```python
from build123d import *

# Parameters (mm, degrees)
F0_W     = 50
F0_H     = 50
F1_DEPTH = 30
F2_R     = 4.45
F3_DEPTH = 30
F3_TAPER = -2
F4_W     = 50
F4_H     = 70
F5_DEPTH = 10


with BuildPart() as f1:
    # F0 (on Top) → F1 (new body)
    with BuildSketch(Plane.XY):
        Rectangle(F0_W, F0_H)
    extrude(amount=F1_DEPTH)

    # F2 (on Top) → F3 (cut)
    with BuildSketch(Plane.XY):
        with Locations((10, 10)):
            Circle(F2_R)
        with Locations((-10, 10)):
            Circle(F2_R)
        with Locations((10, -10)):
            Circle(F2_R)
        with Locations((-10, -10)):
            Circle(F2_R)
    extrude(amount=F3_DEPTH, taper=F3_TAPER, mode=Mode.SUBTRACT)

    # F4 (on Top) → F5 (join)
    with BuildSketch(Plane.XY):
        Rectangle(F4_W, F4_H)
    extrude(amount=-F5_DEPTH)


solid = f1.part
```
Geometry check sheet. Reference: the model listing, model coordinates, mm. A direction names the side the tool comes from. Coordinates: 2 decimals unless noted, no trailing zeros. Order: outer loops, then holes, each group sorted by start corner. A loop starts at its lowest first (then second) coordinate and runs counter-clockwise, first axis right, second up.
Q1. Tool access check on faces 1 (the face through (0, 0, -10)), 2 (the face through (0, 35, -5)), 3 (the face through (0, -30, 0)), 4 (the face through (0, 30, 0)), 5 (the face through (10, -10, 0)). Record the directions out of +Z, -Z, +X, -X, +Y, -Y that give a thin tool (end or side, any length) a straight path to the whole face; none if there is none.
Reply:
face 1: -Z, +X, -X, +Y, -Y
face 2: +Z, -Z, +X, -X, +Y
face 3: +Z, +X, -X, -Y
face 4: +Z, +X, -X, +Y
face 5: +Z
Q2. Thickness scan on probe 1 along Y at (x, z) = (-10, 27); probe 2 along Y at (x, z) = (12.5, 21.5); probe 3 along X at (y, z) = (-5.5, 28). Record the ranges inside material, lowest first.
Reply:
probe 1: y = -25 to -15.39, -4.61 to 4.61, 15.39 to 25
probe 2: y = -25 to -14.56, -5.44 to 5.44, 14.56 to 25
probe 3: x = -25 to -13.03, -6.97 to 6.97, 13.03 to 25
Q3. Sectioned sample at A-A on x = 0.5. Record the cut outline in (y, z).
Reply:
outline: (-35, -10) - (35, -10) - (35, 0) - (25, 0) - (25, 30) - (-25, 30) - (-25, 0) - (-35, 0) - close
Q4. Sectioned sample at B-B on z = 26. Record the cut outline in (x, y), and give its area (3 significant figures).
Reply:
outline: (-25, -25) - (25, -25) - (25, 25) - (-25, 25) - close; hole circle Ø10.72 at (-10, -10); hole circle Ø10.72 at (-10, 10); hole circle Ø10.72 at (10, -10); hole circle Ø10.72 at (10, 10)
area: 2,140 mm2
Q5. Sectioned sample at D-D on x = -10. Record the cut outline in (y, z), and give its area (3 significant figures).
Reply:
outline: (-35, -10) - (35, -10) - (35, 0) - (25, 0) - (25, 30) - (15.5, 30) - (14.45, 0) - (5.55, 0) - (4.5, 30) - (-4.5, 30) - (-5.55, 0) - (-14.45, 0) - (-15.5, 30) - (-25, 30) - (-25, 0) - (-35, 0) - close
area: 1,600 mm2
Q6. Draft check along X on faces 6 (the face through (25, 0, 10)), 7 (the face through (-5.25, -8.5, 15.21)), 8 (the face through (10, 10, 0)), 9 (the face through (0, -35, -5)). Enter one of: released by +X, released by -X, zero draft, split by the parting line, or undercut.
Reply:
face 6: released by +X
face 7: undercut
face 8: undercut
face 9: zero draft
Q7. Depth check by flat-ended pin: pin 1 Ø12 at (x, z) = (3, 9) entering from -Y; pin 2 Ø2 at (x, z) = (8, 21) entering from +Y; pin 3 Ø2.5 at (x, y) = (-12, 9) entering from +Z. Enter the tip coordinate at first touch or a pass-through.
Reply:
pin 1: stops at y = -25
pin 2: stops at y = 25
pin 3: stops at z = 0
Q8. Sectioned sample at C-C on y = 31. Record the cut outline in (x, z).
Reply:
outline: (-25, -10) - (25, -10) - (25, 0) - (-25, 0) - close
